```python
from build123d import *

# Parameters (mm, degrees)
SKETCH1_W           = 88.9
SKETCH1_H           = 46.99
SKETCH1_R           = 1.905
BOSS_EXTRUDE1_DEPTH = 3.175


with BuildPart() as part:
    # Sketch1 → Boss-Extrude1 (new body)
    with BuildSketch(Plane.XY):
        with Locations((80.175941247, 30.1625)):
            Rectangle(SKETCH1_W, SKETCH1_H)
        with Locations((48.77435, 49.2125)):
            Circle(SKETCH1_R, mode=Mode.SUBTRACT)
        with Locations((111.56315, 49.2125)):
            Circle(SKETCH1_R, mode=Mode.SUBTRACT)
        with Locations((48.77435, 11.1125)):
            Circle(SKETCH1_R, mode=Mode.SUBTRACT)
        with Locations((111.56315, 11.1125)):
            Circle(SKETCH1_R, mode=Mode.SUBTRACT)
        with BuildLine():
            ThreePointArc((83.469406447, 24.4520759), (80.069406447, 27.8520759), (76.669406447, 24.4520759))
            ThreePointArc((76.669406447, 24.4520759), (80.069406447, 21.0520759), (83.469406447, 24.4520759))
        make_face(mode=Mode.SUBTRACT)
        with BuildLine():
            ThreePointArc((106.780920888, 36.184870981), (110.180920888, 32.784870981), (113.580920888, 36.184870981))
            ThreePointArc((113.580920888, 36.184870981), (110.180920888, 39.584870981), (106.780920888, 36.184870981))
        make_face(mode=Mode.SUBTRACT)
        with BuildLine():
            ThreePointArc((53.381968416, 35.458841184), (49.600968416, 39.239841184), (45.819968416, 35.458841184))
            ThreePointArc((45.819968416, 35.458841184), (49.600968416, 31.677841184), (53.381968416, 35.458841184))
        make_face(mode=Mode.SUBTRACT)
        with BuildLine():
            ThreePointArc((83.689808954, 42.509614322), (79.908808954, 46.290614322), (76.127808954, 42.509614322))
            ThreePointArc((76.127808954, 42.509614322), (79.908808954, 38.728614322), (83.689808954, 42.509614322))
        make_face(mode=Mode.SUBTRACT)
    extrude(amount=BOSS_EXTRUDE1_DEPTH)


solid = part.part
```
The listing builds one solid part. Answer for the finished solid, in the listing's coordinates (mm). Round coordinates to 2 decimals unless told otherwise and drop trailing zeros. Loops run counter-clockwise (first coordinate to the right, second up) from the corner with the lowest first, then second, coordinate; pieces in that order, holes last.
1) For a pull along Y with two mould halves and no side action, classify faces 1 (the face through (80, 6.668, 2)), 2 (the face through (50.591, 49.785, 1.565)), 3 (the face through (35.726, 30, 2)), 4 (the face through (50.534, 10.383, 1.565)) as released by +Y, released by -Y, zero draft, split by the parting line, or undercut.
Outcome:
face 1: released by -Y
face 2: undercut
face 3: zero draft
face 4: undercut
2) A cutting plane is placed at B-B on y = 23.5. Determine the outline of the cut face in (x, z) (3 decimals), plus the area to 3 significant figures.
Outcome:
outline: (35.726, 0) - (76.805, 0) - (76.805, 3.175) - (35.726, 3.175) - close; (83.333, 0) - (124.626, 0) - (124.626, 3.175) - (83.333, 3.175) - close
area: 262 mm2
3) A cutting plane is placed at A-A on x = 77.5. Determine the outline of the cut face in (y, z) (1 decimal).
Outcome:
outline: (6.7, 0) - (22.2, 0) - (22.2, 3.2) - (6.7, 3.2) - close; (26.7, 0) - (39.6, 0) - (39.6, 3.2) - (26.7, 3.2) - close; (45.4, 0) - (53.7, 0) - (53.7, 3.2) - (45.4, 3.2) - close
4) A cutting plane is placed at C-C on z = 0.8. Give the number of separate pieces and of enclosed holes in the cut face, plus the area to 3 significant figures.
Outcome:
separate pieces: 1
enclosed holes: 8
area: 3,970 mm2
5) Consider line 1 (Y direction, x = 80, z = 2); line 2 (X direction, y = 35, z = 2.8); line 3 (X direction, y = 48, z = 2.4). Determine where each line is inside the solid, lowest interval first.
Outcome:
line 1: y = 6.67 to 21.05, 27.85 to 38.73, 46.29 to 53.66
line 2: x = 35.73 to 45.85, 53.35 to 106.99, 113.37 to 124.63
line 3: x = 35.73 to 47.31, 50.24 to 110.09, 113.03 to 124.63
